```python
from build123d import *

# Parameters (mm, degrees)
SKETCH1_R           = 5.65
BOSS_EXTRUDE1_DEPTH = 7
SKETCH2_R           = 5.65
BOSS_EXTRUDE2_DEPTH = 14.74
SKETCH3_R           = 5.65
BOSS_EXTRUDE3_DEPTH = 14


with BuildPart() as part:
    # Sketch1 → Boss-Extrude1 (new body)
    # profile 1 of 12: a face of its own
    with BuildSketch(Plane.XY):
        Circle(SKETCH1_R)
        with BuildLine():
            ThreePointArc((-0.81964124, -3.557591308), (-1.028546403, -3.50290736), (-1.233852984, -3.435967766))
            ThreePointArc((-1.233852984, -3.435967766), (-1.973766094, -3.071239991), (-2.612905161, -2.549704746))
            ThreePointArc((-2.612905161, -2.549704746), (-2.759082994, -2.390759024), (-2.895607604, -2.223448736))
            ThreePointArc((-2.895607604, -2.223448736), (-3.320875399, -1.516592978), (-3.576590156, -0.732304943))
            ThreePointArc((-3.576590156, -0.732304943), (-3.613630229, -0.519561589), (-3.638027269, -0.305000442))
            ThreePointArc((-3.638027269, -0.305000442), (-3.613630229, 0.519561589), (-3.404733048, 1.317596505))
            ThreePointArc((-3.404733048, 1.317596505), (-3.320875399, 1.516592978), (-3.225398981, 1.710283337))
            ThreePointArc((-3.225398981, 1.710283337), (-2.759082994, 2.390759024), (-2.151897253, 2.949170373))
            ThreePointArc((-2.151897253, 2.949170373), (-1.973766094, 3.071239991), (-1.788729306, 3.182564241))
            ThreePointArc((-1.788729306, 3.182564241), (-1.028546403, 3.50290736), (-0.215849285, 3.644403485))
            ThreePointArc((-0.215849285, 3.644403485), (-0.107971873, 3.649193027), (0, 3.650790007))
            ThreePointArc((0, 3.650790007), (0.107971873, 3.649193027), (0.215849285, 3.644403485))
            ThreePointArc((0.215849285, 3.644403485), (1.028546403, 3.50290736), (1.788729306, 3.182564241))
            ThreePointArc((1.788729306, 3.182564241), (1.973766094, 3.071239991), (2.151897253, 2.949170373))
            ThreePointArc((2.151897253, 2.949170373), (2.759082994, 2.390759024), (3.225398981, 1.710283337))
            ThreePointArc((3.225398981, 1.710283337), (3.320875399, 1.516592978), (3.404733048, 1.317596505))
            ThreePointArc((3.404733048, 1.317596505), (3.588748603, 0.670187395), (3.650790007, 0))
            ThreePointArc((3.650790007, 0), (3.647597927, -0.152633677), (3.638027269, -0.305000442))
            ThreePointArc((3.638027269, -0.305000442), (3.613630229, -0.519561589), (3.576590156, -0.732304943))
            ThreePointArc((3.576590156, -0.732304943), (3.320875399, -1.516592978), (2.895607604, -2.223448736))
            ThreePointArc((2.895607604, -2.223448736), (2.759082994, -2.390759024), (2.612905161, -2.549704746))
            ThreePointArc((2.612905161, -2.549704746), (1.973766094, -3.071239991), (1.233852984, -3.435967766))
            ThreePointArc((1.233852984, -3.435967766), (1.028546403, -3.50290736), (0.81964124, -3.557591308))
            ThreePointArc((0.81964124, -3.557591308), (0, -3.650790007), (-0.81964124, -3.557591308))
        make_face(mode=Mode.SUBTRACT)
    # profile 2 of 12: a face of its own
    with BuildSketch(Plane.XY):
        with BuildLine():
            ThreePointArc((-2.151897253, 2.949170373), (-2.759082994, 2.390759024), (-3.225398981, 1.710283337))
            ThreePointArc((-3.225398981, 1.710283337), (-2.902782795, 1.721509121), (-2.585426091, 1.662416447))
            ThreePointArc((-2.585426091, 1.662416447), (-2.562741672, 1.6561643), (-2.539777266, 1.651035136))
            ThreePointArc((-2.539777266, 1.651035136), (-2.085465777, 1.807066382), (-1.99567797, 2.278959198))
            ThreePointArc((-1.99567797, 2.278959198), (-2.004023102, 2.300959902), (-2.013439941, 2.322523654))
            ThreePointArc((-2.013439941, 2.322523654), (-2.117095704, 2.628240359), (-2.151897253, 2.949170373))
        make_face()
    # profile 3 of 12: a face of its own
    with BuildSketch(Plane.XY):
        with BuildLine():
            ThreePointArc((-0.215849285, 3.644403485), (-1.028546403, 3.50290736), (-1.788729306, 3.182564241))
            ThreePointArc((-1.788729306, 3.182564241), (-1.511258183, 3.017588493), (-1.276228646, 2.796300584))
            ThreePointArc((-1.276228646, 2.796300584), (-1.260525464, 2.77877682), (-1.243979612, 2.762046398))
            ThreePointArc((-1.243979612, 2.762046398), (-0.777431606, 2.6476889), (-0.446772779, 2.996127445))
            ThreePointArc((-0.446772779, 2.996127445), (-0.441898672, 3.019147334), (-0.438162377, 3.042379044))
            ThreePointArc((-0.438162377, 3.042379044), (-0.360080224, 3.355604839), (-0.215849285, 3.644403485))
        make_face()
    # profile 4 of 12: a face of its own
    with BuildSketch(Plane.XY):
        with BuildLine():
            ThreePointArc((1.788729306, 3.182564241), (1.028546403, 3.50290736), (0.215849285, 3.644403485))
            ThreePointArc((0.215849285, 3.644403485), (0.360080224, 3.355604839), (0.438162377, 3.042379044))
            ThreePointArc((0.438162377, 3.042379044), (0.441898672, 3.019147334), (0.446772779, 2.996127445))
            ThreePointArc((0.446772779, 2.996127445), (0.777431606, 2.6476889), (1.243979612, 2.762046398))
            ThreePointArc((1.243979612, 2.762046398), (1.260525464, 2.77877682), (1.276228646, 2.796300584))
            ThreePointArc((1.276228646, 2.796300584), (1.511258183, 3.017588493), (1.788729306, 3.182564241))
        make_face()
    # profile 5 of 12: a face of its own
    with BuildSketch(Plane.XY):
        with BuildLine():
            ThreePointArc((2.585426091, 1.662416447), (2.902782795, 1.721509121), (3.225398981, 1.710283337))
            ThreePointArc((3.225398981, 1.710283337), (2.759082994, 2.390759024), (2.151897253, 2.949170373))
            ThreePointArc((2.151897253, 2.949170373), (2.117095704, 2.628240359), (2.013439941, 2.322523654))
            ThreePointArc((2.013439941, 2.322523654), (2.004023102, 2.300959902), (1.99567797, 2.278959198))
            ThreePointArc((1.99567797, 2.278959198), (2.085465777, 1.807066382), (2.539777266, 1.651035136))
            ThreePointArc((2.539777266, 1.651035136), (2.562741672, 1.6561643), (2.585426091, 1.662416447))
        make_face()
    # profile 6 of 12: a face of its own
    with BuildSketch(Plane.XY):
        with BuildLine():
            ThreePointArc((3.07376902, 0.000726834), (3.372694379, -0.121137234), (3.638027269, -0.305000442))
            ThreePointArc((3.638027269, -0.305000442), (3.647597927, -0.152633677), (3.650790007, 0))
            ThreePointArc((3.650790007, 0), (3.588748603, 0.670187395), (3.404733048, 1.317596505))
            ThreePointArc((3.404733048, 1.317596505), (3.201948257, 1.066428135), (2.94946455, 0.865283413))
            ThreePointArc((2.94946455, 0.865283413), (2.929884357, 0.852233959), (2.910969506, 0.838237507))
            ThreePointArc((2.910969506, 0.838237507), (2.731379298, 0.392713056), (3.029213584, 0.015831883))
            ThreePointArc((3.029213584, 0.015831883), (3.051305506, 0.007731316), (3.07376902, 0.000726834))
        make_face()
    # profile 7 of 12: a face of its own
    with BuildSketch(Plane.XY):
        with BuildLine():
            ThreePointArc((2.586212003, -1.661193544), (2.771799329, -1.925323372), (2.895607604, -2.223448736))
            ThreePointArc((2.895607604, -2.223448736), (3.320875399, -1.516592978), (3.576590156, -0.732304943))
            ThreePointArc((3.576590156, -0.732304943), (3.270204862, -0.833967486), (2.949055004, -0.866678197))
            ThreePointArc((2.949055004, -0.866678197), (2.92552803, -0.867070245), (2.902048792, -0.868618669))
            ThreePointArc((2.902048792, -0.868618669), (2.510099192, -1.146323891), (2.556895991, -1.62439788))
            ThreePointArc((2.556895991, -1.62439788), (2.571101401, -1.643156306), (2.586212003, -1.661193544))
        make_face()
    # profile 8 of 12: a face of its own
    with BuildSketch(Plane.XY):
        with BuildLine():
            ThreePointArc((1.277550948, -2.79569671), (1.290877576, -3.118232944), (1.233852984, -3.435967766))
            ThreePointArc((1.233852984, -3.435967766), (1.973766094, -3.071239991), (2.612905161, -2.549704746))
            ThreePointArc((2.612905161, -2.549704746), (2.300194531, -2.469584323), (2.012341335, -2.323475602))
            ThreePointArc((2.012341335, -2.323475602), (1.992337228, -2.311085771), (1.971748095, -2.299694554))
            ThreePointArc((1.971748095, -2.299694554), (1.491880328, -2.321411101), (1.272781988, -2.748892795))
            ThreePointArc((1.272781988, -2.748892795), (1.274590768, -2.772353412), (1.277550948, -2.79569671))
        make_face()
    # profile 9 of 12: a face of its own
    with BuildSketch(Plane.XY):
        with BuildLine():
            ThreePointArc((-0.436723505, -3.042585922), (-0.599888686, -3.321125588), (-0.81964124, -3.557591308))
            ThreePointArc((-0.81964124, -3.557591308), (0, -3.650790007), (0.81964124, -3.557591308))
            ThreePointArc((0.81964124, -3.557591308), (0.599888686, -3.321125588), (0.436723505, -3.042585922))
            ThreePointArc((0.436723505, -3.042585922), (0.426593428, -3.021347897), (0.415431304, -3.00063367))
            ThreePointArc((0.415431304, -3.00063367), (0, -2.75946669), (-0.415431304, -3.000633669))
            ThreePointArc((-0.415431304, -3.000633669), (-0.426593428, -3.021347896), (-0.436723505, -3.042585922))
        make_face()
    # profile 10 of 12: a face of its own
    with BuildSketch(Plane.XY):
        with BuildLine():
            ThreePointArc((-1.233852984, -3.435967766), (-1.290877576, -3.118232944), (-1.277550949, -2.79569671))
            ThreePointArc((-1.277550949, -2.79569671), (-1.274590768, -2.772353411), (-1.272781988, -2.748892794))
            ThreePointArc((-1.272781988, -2.748892794), (-1.491880327, -2.321411102), (-1.971748091, -2.299694555))
            ThreePointArc((-1.971748091, -2.299694555), (-1.992337225, -2.311085772), (-2.012341332, -2.323475603))
            ThreePointArc((-2.012341332, -2.323475603), (-2.300194529, -2.469584324), (-2.612905161, -2.549704746))
            ThreePointArc((-2.612905161, -2.549704746), (-1.973766094, -3.071239991), (-1.233852984, -3.435967766))
        make_face()
    # profile 11 of 12: a face of its own
    with BuildSketch(Plane.XY):
        with BuildLine():
            ThreePointArc((-3.576590156, -0.732304943), (-3.320875399, -1.516592978), (-2.895607604, -2.223448736))
            ThreePointArc((-2.895607604, -2.223448736), (-2.771799329, -1.925323372), (-2.586212003, -1.661193544))
            ThreePointArc((-2.586212003, -1.661193544), (-2.571101401, -1.643156306), (-2.556895991, -1.62439788))
            ThreePointArc((-2.556895991, -1.62439788), (-2.510099192, -1.146323891), (-2.902048792, -0.868618669))
            ThreePointArc((-2.902048792, -0.868618669), (-2.92552803, -0.867070245), (-2.949055004, -0.866678197))
            ThreePointArc((-2.949055004, -0.866678197), (-3.270204862, -0.833967486), (-3.576590156, -0.732304943))
        make_face()
    # profile 12 of 12: a face of its own
    with BuildSketch(Plane.XY):
        with BuildLine():
            ThreePointArc((-3.404733048, 1.317596505), (-3.613630229, 0.519561589), (-3.638027269, -0.305000442))
            ThreePointArc((-3.638027269, -0.305000442), (-3.372694379, -0.121137234), (-3.07376902, 0.000726834))
            ThreePointArc((-3.07376902, 0.000726834), (-3.051305506, 0.007731316), (-3.029213584, 0.015831883))
            ThreePointArc((-3.029213584, 0.015831883), (-2.731379298, 0.392713056), (-2.910969506, 0.838237507))
            ThreePointArc((-2.910969506, 0.838237507), (-2.929884357, 0.852233959), (-2.94946455, 0.865283413))
            ThreePointArc((-2.94946455, 0.865283413), (-3.201948257, 1.066428135), (-3.404733048, 1.317596505))
        make_face()
    extrude(amount=BOSS_EXTRUDE1_DEPTH)

    # Sketch2 → Boss-Extrude2 (add)
    with BuildSketch(Plane.XY.offset(7)):
        Circle(SKETCH2_R)
    extrude(amount=BOSS_EXTRUDE2_DEPTH)

    # Sketch3 → Boss-Extrude3 (add)
    with BuildSketch(Plane.XY.offset(21.74)):
        Circle(SKETCH3_R)
        with BuildLine():
            Line((-1.658312395, 2.5), (1.658312395, 2.5))
            ThreePointArc((1.658312395, 2.5), (0, -3), (-1.658312395, 2.5))
        make_face(mode=Mode.SUBTRACT)
    extrude(amount=BOSS_EXTRUDE3_DEPTH)


solid = part.part
```
Check sheet for the modelled part. Datum: model origin and axes. Units: mm. A direction names the side the tool comes from. Round coordinates to 2 decimals unless told otherwise and drop trailing zeros. Write each loop counter-clockwise with the first axis right and the second up, starting at its lowest first coordinate (ties: lowest second). Pieces come first, ordered by that corner, then holes. Notation, with made-up numbers: (53.5, 38) -> (85.5, 38) arc R13 cw to (85.5, 62) -> close; hole circle Ø2 at (21.5, -4). An arc over 180 degrees is marked (long way). Put each result on its own line as item: value.
(1) Sectioned sample at A-A (z = 9). Enter the section's corners in (x, y), plus the area to 3 significant figures.
Values found:
outline: circle Ø11.3 at (0, 0)
area: 100 mm^2
(2) Go/stop test with flat-tipped pins: pin 1 Ø1.5 at (x, y) = (-1.5, -1) entering from -Z; pin 2 Ø6 at (y, z) = (-4, 13.5) entering from -X; pin 3 Ø6 at (y, z) = (4.5, 16) entering from -X. Record where each tip stops, or that it passes through.
Values found:
pin 1: stops at z = 7
pin 2: stops at x = -5.56
pin 3: stops at x = -5.45
(3) Tool access check on faces 4 (the face through (0, 2.5, 29)), 5 (the face through (0, 0, 7)), 6 (the face through (0, 3, 35.74)). Record the directions out of +Z, -Z, +X, -X, +Y, -Y that give a thin tool (end or side, any length) a straight path to the whole face; none if there is none.
Values found:
face 4: +Z
face 5: -Z
face 6: +Z, +X, -X, +Y, -Y
(4) Material ranges on line 1 (Y direction, x = 0, z = 28); line 2 (X direction, y = -3.25, z = 5.5); line 3 (Z direction, x = -1.25, y = 2.25), recorded low to high.
Values found:
line 1: y = -5.65 to -3, 2.5 to 5.65
line 2: x = -4.62 to -1.28, -0.55 to 0.55, 1.28 to 4.62
line 3: z = 7 to 21.74
(5) Mould release check, pull along Y, two halves, no side actions. Record for faces 1 (the face through (5.39, 1.7, 17.62)), 2 (the face through (2.4, 2.6, 0)), 3 (the face through (0, 0, 21.74)): released by +Y, released by -Y, zero draft, split by the parting line, or undercut.
Values found:
face 1: split by the parting line
face 2: zero draft
face 3: undercut
